For this review, take the finished solid that the model builds, in its own axes (mm). Coordinates: 2 decimals unless noted, no trailing zeros.
Autodesk Inventor part; units mm, degrees
ref_plane "YZ Plane" through (0, 0, 0) normal (1, 0, 0) x (0, 1, 0)
ref_plane "XZ Plane" through (0, 0, 0) normal (0, 1, 0) x (-1, 0, 0)
ref_plane "XY Plane" through (0, 0, 0) normal (0, 0, 1) x (1, 0, 0)
sketch "Sketch1" plane through (0, 0, 0) normal (0, 0, 1) x (1, 0, 0)
  line L0 (-8, -10) -> (-3.2, -10)
  arc A0 (-10, -8) -> (-8, -10) centre (-8, -8) ccw
  line L1 (3.2, -10) -> (8, -10)
  line L2 (-8, 10) -> (-3.2, 10)
  line L3 (3.2, 10) -> (8, 10)
  line L4 (-10, 8) -> (-10, 3.2)
  arc A1 (-8, 10) -> (-10, 8) centre (-8, 8) ccw
  line L5 (-10, -3.2) -> (-10, -8)
  line L6 (10, 8) -> (10, 3.2)
  arc A2 (10, 8) -> (8, 10) centre (8, 8) ccw
  line L7 (10, -3.2) -> (10, -8)
  arc A3 (8, -10) -> (10, -8) centre (8, -8) ccw
  circle A4 centre (0, 0) radius 2.6
  line L8 (8.65, 4.6) -> (8.65, 3.2)
  line L9 (8.65, -3.2) -> (8.65, -4.6)
  arc A5 (8.15, -5.1) -> (8.65, -4.6) centre (8.15, -4.6) ccw
  arc A6 (8.65, 4.6) -> (8.15, 5.1) centre (8.15, 4.6) ccw
  line L10 (3.9, 2.0109) -> (3.9, -2.0109)
  arc A7 (4.4858, 3.4251) -> (3.9, 2.0109) centre (5.9, 2.0109) ccw
  line L11 (8.65, 3.2) -> (10, 3.2)
  line L12 (8.65, -3.2) -> (10, -3.2)
  line L13 (6.3678, -5.1) -> (8.15, -5.1)
  arc A8 (6.0142, -4.9536) -> (6.3678, -5.1) centre (6.3678, -4.6) ccw
  line L14 (6.3678, 5.1) -> (8.15, 5.1)
  arc A9 (6.3678, 5.1) -> (6.0142, 4.9536) centre (6.3678, 4.6) ccw
  line L15 (4.4858, 3.4251) -> (6.0142, 4.9536)
  line L16 (4.4858, -3.4251) -> (6.0142, -4.9536)
  arc A10 (3.9, -2.0109) -> (4.4858, -3.4251) centre (5.9, -2.0109) ccw
  line L17 (-4.6, 8.65) -> (-3.2, 8.65)
  line L18 (3.2, 8.65) -> (4.6, 8.65)
  arc A11 (5.1, 8.15) -> (4.6, 8.65) centre (4.6, 8.15) ccw
  arc A12 (-4.6, 8.65) -> (-5.1, 8.15) centre (-4.6, 8.15) ccw
  line L19 (-2.0109, 3.9) -> (2.0109, 3.9)
  arc A13 (-3.4251, 4.4858) -> (-2.0109, 3.9) centre (-2.0109, 5.9) ccw
  line L20 (-3.2, 8.65) -> (-3.2, 10)
  line L21 (3.2, 8.65) -> (3.2, 10)
  line L22 (5.1, 6.3678) -> (5.1, 8.15)
  arc A14 (4.9536, 6.0142) -> (5.1, 6.3678) centre (4.6, 6.3678) ccw
  line L23 (-5.1, 6.3678) -> (-5.1, 8.15)
  arc A15 (-5.1, 6.3678) -> (-4.9536, 6.0142) centre (-4.6, 6.3678) ccw
  line L24 (-3.4251, 4.4858) -> (-4.9536, 6.0142)
  line L25 (3.4251, 4.4858) -> (4.9536, 6.0142)
  arc A16 (2.0109, 3.9) -> (3.4251, 4.4858) centre (2.0109, 5.9) ccw
  line L26 (-8.65, -4.6) -> (-8.65, -3.2)
  line L27 (-8.65, 3.2) -> (-8.65, 4.6)
  arc A17 (-8.15, 5.1) -> (-8.65, 4.6) centre (-8.15, 4.6) ccw
  arc A18 (-8.65, -4.6) -> (-8.15, -5.1) centre (-8.15, -4.6) ccw
  line L28 (-3.9, -2.0109) -> (-3.9, 2.0109)
  arc A19 (-4.4858, -3.4251) -> (-3.9, -2.0109) centre (-5.9, -2.0109) ccw
  line L29 (-8.65, -3.2) -> (-10, -3.2)
  line L30 (-8.65, 3.2) -> (-10, 3.2)
  line L31 (-6.3678, 5.1) -> (-8.15, 5.1)
  arc A20 (-6.0142, 4.9536) -> (-6.3678, 5.1) centre (-6.3678, 4.6) ccw
  line L32 (-6.3678, -5.1) -> (-8.15, -5.1)
  arc A21 (-6.3678, -5.1) -> (-6.0142, -4.9536) centre (-6.3678, -4.6) ccw
  line L33 (-4.4858, -3.4251) -> (-6.0142, -4.9536)
  line L34 (-4.4858, 3.4251) -> (-6.0142, 4.9536)
  arc A22 (-3.9, 2.0109) -> (-4.4858, 3.4251) centre (-5.9, 2.0109) ccw
  line L35 (4.6, -8.65) -> (3.2, -8.65)
  line L36 (-3.2, -8.65) -> (-4.6, -8.65)
  arc A23 (-5.1, -8.15) -> (-4.6, -8.65) centre (-4.6, -8.15) ccw
  arc A24 (4.6, -8.65) -> (5.1, -8.15) centre (4.6, -8.15) ccw
  line L37 (2.0109, -3.9) -> (-2.0109, -3.9)
  arc A25 (3.4251, -4.4858) -> (2.0109, -3.9) centre (2.0109, -5.9) ccw
  line L38 (3.2, -8.65) -> (3.2, -10)
  line L39 (-3.2, -8.65) -> (-3.2, -10)
  line L40 (-5.1, -6.3678) -> (-5.1, -8.15)
  arc A26 (-4.9536, -6.0142) -> (-5.1, -6.3678) centre (-4.6, -6.3678) ccw
  line L41 (5.1, -6.3678) -> (5.1, -8.15)
  arc A27 (5.1, -6.3678) -> (4.9536, -6.0142) centre (4.6, -6.3678) ccw
  line L42 (3.4251, -4.4858) -> (4.9536, -6.0142)
  line L43 (-3.4251, -4.4858) -> (-4.9536, -6.0142)
  arc A28 (-2.0109, -3.9) -> (-3.4251, -4.4858) centre (-2.0109, -5.9) ccw
  dimension "d0" = 0.5
  dimension "d1" = 2
  dimension "d2" = 5.2
  dimension "d3" = 45
  dimension "d4" = 45
  dimension "d5" = 45
  dimension "d6" = 90
  dimension "d7" = 90
  dimension "d8" = 45
  dimension "d9" = 45
  dimension "d10" = 90
  dimension "d11" = 90
  dimension "d12" = 90
  dimension "d13" = 90
  dimension "d14" = 90
  dimension "d15" = 90
  dimension "d16" = 90
  dimension "d17" = 90
  dimension "d18" = 90
  dimension "d19" = 90
  dimension "d20" = 90
  dimension "d21" = 90
  dimension "d22" = 90
  dimension "d23" = 90
  dimension "d24" = 1.35
  dimension "d25" = 4.9
  dimension "d26" = 6.1
  dimension "d27" = 6.8
  dimension "d28" = 13.2
  dimension "d29" = 13.9
  dimension "d30" = 15.1
  dimension "d31" = 18.65
  dimension "d32" = 20
  dimension "d33" = 6.4
  dimension "d34" = 1.9
  dimension "d35" = 8.3
  dimension "d36" = 6.8
  dimension "d37" = 13.2
  dimension "d38" = 5.45
  dimension "d39" = 11.85
  dimension "d40" = 0.7
  dimension "d41" = 7.1
  dimension "d42" = 1.5
  dimension "d43" = 1.5
  dimension "d44" = 10
  dimension "d45" = 10
  dimension "d46" = 3.2
  dimension "d47" = 8.65
  dimension "d48" = 0.75
  dimension "d49" = 0.75
  dimension "d50" = 5.1
  dimension "d51" = 0.75
  dimension "d52" = 3.2
  dimension "d53" = 3.2
  dimension "d54" = 8.65
  dimension "d55" = 8.65
  dimension "d56" = 0.75
  dimension "d57" = 0.75
  dimension "d58" = 5.1
  dimension "d59" = 0.75
  dimension "d60" = 10
  dimension "d61" = 10
  dimension "d62" = 5.1
  dimension "d63" = 5.1
extrude "Extrusion1" add sketch "Sketch1" along normal mid plane 335
equation "\"platform_width\" = 214"
equation "\"platform_depth\" = 214"
equation "\"bed_cl_y_offset\" = 173.25"
properties part number "2020 Extrusion - Double Z motor - Bed X" material "Aluminum 6061"
1. The part is to be moulded in two halves that separate along Y. For faces 1 (the face through (2, 2, -167.5)), 2 (the face through (-0.338, -2.578, -2.345)), say which applies: +Y half, -Y half, draft (parallel to the pull), parting line (faces both ways), or undercut.
Answer below:
face 1: draft
face 2: undercut
2. To check wall thickness, follow L1, parallel to X at y = -6.25, z = -30.5; L2, parallel to Y at x = 0, z = -51; L3, parallel to Y at x = -4.25, z = -84.5. State the ranges of each line that lie inside material, in increasing order.
Answer below:
L1: x = -10 to -5.09, 5.09 to 10
L2: y = -3.9 to -2.6, 2.6 to 3.9
L3: y = -10 to -8.65, -5.31 to -3.14, 3.14 to 5.31, 8.65 to 10
3. Clearance check with flat-ended pins moving along their axes: pin 1 Ø4.5 at (x, y) = (0, 0) entering from -Z; pin 2 Ø1.5 at (y, z) = (9.5, -65.5) entering from -X; pin 3 Ø1.5 at (y, z) = (9, -26) entering from +X; pin 4 Ø1.2 at (y, z) = (-0.5, -6.5) entering from +X. State where each tip first meets the part, or that it passes through.
Answer below:
pin 1: passes through
pin 2: stops at x = -9.85
pin 3: stops at x = 9.98
pin 4: stops at x = 3.9
